from build123d import *

# Parameters (mm, degrees)
SKETCH_1_W          = 29.4
SKETCH_1_H          = 19.4
SKETCH_1_W_2        = 23.4
SKETCH_1_H_2        = 13.4
EXTRUDE_1_DEPTH     = 16.4
SKETCH_2_W          = 29.4
SKETCH_2_H          = 19.4
EXTRUDE_2_DEPTH     = 0.8
SKETCH_7_W          = 13.4
SKETCH_7_H          = 5.6
CUT_EXTRUDE_2_DEPTH = 30
SKETCH_8_W          = 23.4
SKETCH_8_H          = 5.6
CUT_EXTRUDE_3_DEPTH = 30
SKETCH_9_W          = 19.4
SKETCH_9_H          = 3
EXTRUDE_5_DEPTH     = 4.2
CUT_EXTRUDE_4_DEPTH = 20.2
CUT_EXTRUDE_5_DEPTH = 5.1
SKETCH_12_R         = 1
CUT_EXTRUDE_6_DEPTH = 2.2
CUT_EXTRUDE_7_DEPTH = 15.4


with BuildPart() as part:
    # 草图1 → 凸台-拉伸1 (new body)
    with BuildSketch(Plane(origin=(0, 0, 0), x_dir=(1, 0, 0), z_dir=(0, 1, 0))):
        Rectangle(SKETCH_1_W, SKETCH_1_H)
        Rectangle(SKETCH_1_W_2, SKETCH_1_H_2, mode=Mode.SUBTRACT)
    extrude(amount=EXTRUDE_1_DEPTH)

    # 草图2 → 凸台-拉伸2 (add)
    with BuildSketch(Plane(origin=(0, 16.4, 0), x_dir=(1, 0, 0), z_dir=(0, 1, 0))):
        Rectangle(SKETCH_2_W, SKETCH_2_H)
    extrude(amount=EXTRUDE_2_DEPTH)

    # 草图7 → 切除-拉伸2 (cut)
    with BuildSketch(Plane.ZY.offset(14.7)):
        with Locations((0, 11.4)):
            Rectangle(SKETCH_7_W, SKETCH_7_H)
        with Locations((0, 5.8)):
            Rectangle(SKETCH_7_W, SKETCH_7_H)
    extrude(amount=-CUT_EXTRUDE_2_DEPTH, mode=Mode.SUBTRACT)

    # 草图8 → 切除-拉伸3 (cut)
    with BuildSketch(Plane(origin=(0, 0, -9.7), x_dir=(-1, 0, 0), z_dir=(0, 0, -1))):
        with Locations((0, 11.4)):
            Rectangle(SKETCH_8_W, SKETCH_8_H)
        with Locations((0, 5.8)):
            Rectangle(SKETCH_8_W, SKETCH_8_H)
    extrude(amount=-CUT_EXTRUDE_3_DEPTH, mode=Mode.SUBTRACT)

    # 草图9 → 凸台-拉伸5 (add)
    with BuildSketch(Plane(origin=(14.7, 0, 0), x_dir=(0, 0, -1), z_dir=(1, 0, 0))):
        with Locations((0, 1.5)):
            Rectangle(SKETCH_9_W, SKETCH_9_H)
    extrude_5 = extrude(amount=EXTRUDE_5_DEPTH)

    # 草图10 → 切除-拉伸4 (cut)
    with BuildSketch(Plane.XY.offset(9.7)):
        with BuildLine():
            add(Edge.make_bspline(
                [(18.486644801, 1.737785066), (18.825886074, 1.616028978), (18.9, 1.36920832)],
                knots=[0.049557912, 0.049557912, 0.049557912, 0.659174515, 0.659174515, 0.659174515], degree=2))
            Line((18.9, 1.36920832), (18.9, 1.6))
            Line((18.9, 1.6), (18.9, 3))
            Line((18.9, 3), (14.7, 3))
            Line((14.7, 3), (18.429736397, 1.756754534))
            add(Edge.make_bspline(
                [(18.429736397, 1.756754534), (18.459066665, 1.747683054), (18.486644801, 1.737785066)],
                knots=[0, 0, 0, 0.049557912, 0.049557912, 0.049557912], degree=2))
        make_face()
    cut_extrude_4 = extrude(amount=-CUT_EXTRUDE_4_DEPTH, mode=Mode.SUBTRACT)

    # 草图11 → 切除-拉伸5 (cut, symmetric)
    with BuildSketch(Plane(origin=(14.7, 0, 0), x_dir=(0, 0, -1), z_dir=(1, 0, 0))):
        Polygon((2.5, 1.3), (6.7, 3), (-6.7, 3), (-2.5, 1.3), align=None)
    cut_extrude_5 = extrude(amount=CUT_EXTRUDE_5_DEPTH, both=True, mode=Mode.SUBTRACT)

    # 草图12 → 切除-拉伸6 (cut)
    with BuildSketch(Plane(origin=(0, 1.3, 0), x_dir=(1, 0, 0), z_dir=(0, 1, 0))):
        with Locations(Location((16.8, 0, 0), (0, 0, 270))):
            Circle(SKETCH_12_R)
    cut_extrude_6 = extrude(amount=-CUT_EXTRUDE_6_DEPTH, mode=Mode.SUBTRACT)

    # 镜向1: 凸台-拉伸5, 切除-拉伸4, 切除-拉伸5, 切除-拉伸6 across plane
    add(extrude_5.mirror(Plane(origin=(0, 0, 0), x_dir=(0, 0, 1), z_dir=(1, 0, 0))))
    add(cut_extrude_4.mirror(Plane(origin=(0, 0, 0), x_dir=(0, 0, 1), z_dir=(1, 0, 0))), mode=Mode.SUBTRACT)
    add(cut_extrude_5.mirror(Plane(origin=(0, 0, 0), x_dir=(0, 0, 1), z_dir=(1, 0, 0))), mode=Mode.SUBTRACT)
    add(cut_extrude_6.mirror(Plane(origin=(0, 0, 0), x_dir=(0, 0, 1), z_dir=(1, 0, 0))), mode=Mode.SUBTRACT)

    # 草图13 → 切除-拉伸7 (cut)
    with BuildSketch(Plane(origin=(0, 17.2, 0), x_dir=(1, 0, 0), z_dir=(0, 1, 0))):
        Polygon((-14.7, 9.7), (14.7, 9.7), (18.9, 9.7), (18.9, 8.2), (14.7, 8.2), (-14.7, 8.2), (-18.9, 8.2), (-18.9, 9.7), align=None)
        Polygon((14.7, -9.7), (-14.7, -9.7), (-18.9, -9.7), (-18.9, -8.2), (-14.7, -8.2), (14.7, -8.2), (18.9, -8.2), (18.9, -9.7), align=None)
    extrude(amount=-CUT_EXTRUDE_7_DEPTH, mode=Mode.SUBTRACT)


solid = part.part
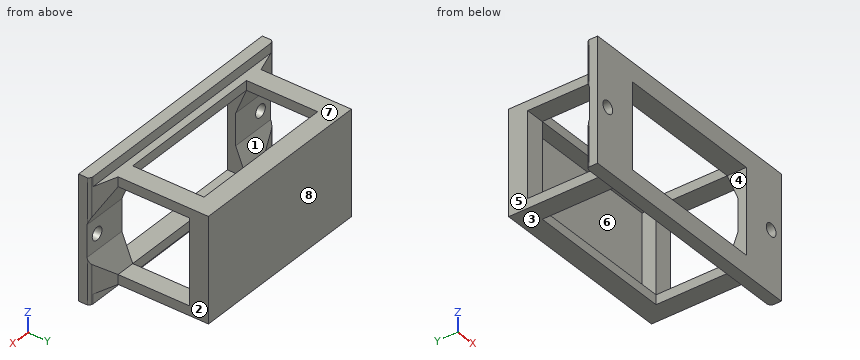
Source: CAD feature listing. Evaluate the final solid. Frame: model axes, mm. Face numbers are marked on the shaded views. A direction names the side the tool comes from. Coordinates: 2 decimals unless noted, no trailing zeros. Loops run counter-clockwise (first coordinate to the right, second up) from the corner with the lowest first, then second, coordinate; pieces in that order, holes last. Notation, with made-up numbers: M 79.5,4 L 97.5,4 A28 cw 97.5,31 Z; hole C -6.5,30 d11. An arc over 180 degrees is marked long. Answer in a Markdown table with one row per item.
Q1. Section B-B on y = 16. Return the cut outline in (x, z), plus the area to 3 significant figures.
Answers below:
| item | result |
|---|---|
| outline | M -14.7,-8.2 L 14.7,-8.2 L 14.7,8.2 L -14.7,8.2 Z; hole M -11.7,-6.7 L 11.7,-6.7 L 11.7,6.7 L -11.7,6.7 Z |
| area | 169 mm^2 |
Q2. Section C-C on x = -11. Return the cut outline in (y, z).
Answers below:
| item | result |
|---|---|
| outline | M 0,-9.7 L 1.8,-9.7 L 1.8,-8.2 L 3,-8.2 L 3,-6.7 L 0,-6.7 Z; M 0,6.7 L 3,6.7 L 3,8.2 L 1.8,8.2 L 1.8,9.7 L 0,9.7 Z; M 14.2,-8.2 L 17.2,-8.2 L 17.2,8.2 L 14.2,8.2 L 14.2,6.7 L 16.4,6.7 L 16.4,-6.7 L 14.2,-6.7 Z |
Q3. Section A-A on z = 0. Return the cut outline in (x, y), plus the area to 3 significant figures.
Answers below:
| item | result |
|---|---|
| outline | M -18.9,0 L -17.8,0 L -17.8,1.3 L -18.9,1.3 Z; M -15.8,0 L -11.7,0 L -11.7,1.3 L -15.8,1.3 Z; M -14.7,14.2 L -11.7,14.2 L -11.7,16.4 L 11.7,16.4 L 11.7,14.2 L 14.7,14.2 L 14.7,17.2 L -14.7,17.2 Z; M 11.7,0 L 15.8,0 L 15.8,1.3 L 11.7,1.3 Z; M 17.8,0 L 18.9,0 L 18.9,1.3 L 17.8,1.3 Z |
| area | 50.2 mm^2 |
Q4. Set-up query: the marked faces 1, 2, 3, 4 and 5. Return all of +Z, -Z, +X, -X, +Y, -Y with unobstructed straight access to the full face (end or side cutting, diameter ignored); none if empty.
Answers below:
| item | result |
|---|---|
| face 1 | +X, -X |
| face 2 | +Z, -Z, +X, +Y |
| face 3 | -Z, +X, -X, +Y |
| face 4 | -Y |
| face 5 | +Z, -Z, -X, +Y |
Q5. Section D-D on y = 8.5. Return the cut outline in (x, z), plus the area to 3 significant figures.
Answers below:
| item | result |
|---|---|
| outline | M -14.7,-8.2 L -11.7,-8.2 L -11.7,-6.7 L -14.7,-6.7 Z; M -14.7,6.7 L -11.7,6.7 L -11.7,8.2 L -14.7,8.2 Z; M 11.7,-8.2 L 14.7,-8.2 L 14.7,-6.7 L 11.7,-6.7 Z; M 11.7,6.7 L 14.7,6.7 L 14.7,8.2 L 11.7,8.2 Z |
| area | 18.0 mm^2 |
Q6. First-contact query: pin 1 (0.7 mm diameter, centred on y = 15, z = 1, fed in from -X); pin 2 (2.5 mm diameter, centred on x = 5.5, y = 15.5, fed in from +Z); pin 3 (1.1 mm diameter, centred on y = 15, z = 3.5, fed in from +X). Flat tips, straight axial feed; report the tip coordinate or a pass-through.
Answers below:
| item | result |
|---|---|
| pin 1 | stops at x = -14.7 |
| pin 2 | stops at z = 8.2 |
| pin 3 | stops at x = 14.7 |
Q7. Ray query, probe 1 along Y at (x, z) = (8, 7); probe 2 along Z at (x, y) = (-16.8, 0.35); probe 3 along X at (y, z) = (0.85, 0). Return the intervals inside material, ascending. Write a range as from..to.
Answers below:
| item | result |
|---|---|
| probe 1 | y = 0..3, 14.2..17.2 |
| probe 2 | z = -9.7..-1, 1..9.7 |
| probe 3 | x = -18.9..-17.8, -15.8..-11.7, 11.7..15.8, 17.8..18.9 |
Q8. Draft query along Z for the marked faces 6, 7 and 8. Return one class per face: pulls with the +Z half, pulls with the -Z half, needs draft (parallel to the pull), parting line crosses it, or undercut.
Answers below:
| item | result |
|---|---|
| face 6 | undercut |
| face 7 | pulls with the +Z half |
| face 8 | needs draft |
